Check sheet for the drawn part. Datum: minimum x, y, z corner. Units: mm. A direction names the side the tool comes from. Round coordinates to 2 decimals unless told otherwise and drop trailing zeros. Write each loop counter-clockwise with the first axis right and the second up, starting at its lowest first coordinate (ties: lowest second). Pieces come first, ordered by that corner, then holes. Notation, with made-up numbers: (23.25, -7) - (41.25, -7) arc R11 ccw to (41.25, 7) - close; hole circle Ø1 at (71.5, 29). An arc over 180 degrees is marked (long way). Answer as a JSON object with one key per item and string values. Group by question number.
1) Set-up check for the marked faces 1, 2 and 3: record each of +Z, -Z, +X, -X, +Y, -Y from which the full face is reachable in a straight line by a thin tool's end or side.
2) Section check C-C (x = 66). Enter the section's corners in (y, z), then the cut area to 3 significant figures.
3) Thickness scan on line 1 (Y direction, x = 42, z = 3.75); line 2 (X direction, y = 7.1, z = 63); line 3 (Y direction, x = 66, z = 5). Record the ranges inside material, lowest first.
4) Section check D-D (y = 71). Enter the section's corners in (x, z).
5) Go/stop test with flat-tipped pins: pin 1 Ø3 at (y, z) = (14, 43) entering from -X; pin 2 Ø4 at (x, y) = (20.5, 42.5) entering from +Z; pin 3 Ø16 at (x, z) = (16, 23.5) entering from -Y; pin 4 Ø6.5 at (x, z) = (5, 103) entering from +Y. Record where each tip stops, or that it passes through.
6) Section check B-B (z = 23). Enter the section's corners in (x, y), then the cut area to 3 significant figures.
7) Section check A-A (y = 14). Enter the section's corners in (x, z).
8) Mould release check, pull along Z, two halves, no side actions. Record for the marked faces 4, 5, 6 and 7: +Z half, -Z half, draft (parallel to the pull), parting line (faces both ways), or undercut.
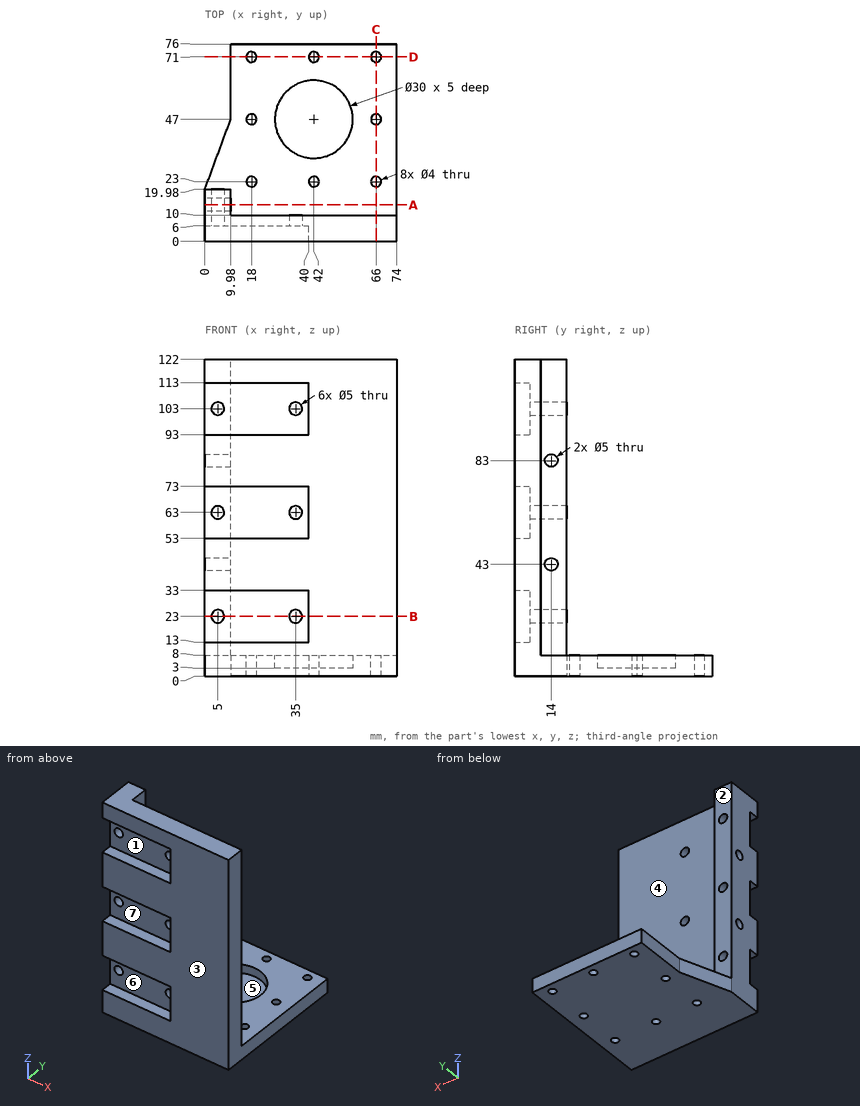
Returned:
{
 "1": {"face 1": "-X, -Y", "face 2": "+Z, +X, -X, +Y", "face 3": "+Z, -Z, +X, -X, -Y"},
 "2": {"outline": "(0, 0) - (21, 0) - (21, 8) - (10, 8) - (10, 122) - (0, 122) - close; (25, 0) - (45, 0) - (45, 8) - (25, 8) - close; (49, 0) - (69, 0) - (69, 8) - (49, 8) - close; (73, 0) - (76, 0) - (76, 8) - (73, 8) - close", "area": "1,650 mm2"},
 "3": {"line 1": "0 to 21, 25 to 32, 62 to 69, 73 to 76", "line 2": "0 to 2.5, 7.5 to 32.5, 37.5 to 74", "line 3": "0 to 21, 25 to 45, 49 to 69, 73 to 76"},
 "4": {"outline": "(9.98, 0) - (16, 0) - (16, 8) - (9.98, 8) - close; (20, 0) - (40, 0) - (40, 8) - (20, 8) - close; (44, 0) - (64, 0) - (64, 8) - (44, 8) - close; (68, 0) - (74, 0) - (74, 8) - (68, 8) - close"},
 "5": {"pin 1": "through", "pin 2": "z = 8", "pin 3": "y = 6", "pin 4": "y = 19.98"},
 "6": {"outline": "(0, 6) - (2.5, 6) - (2.5, 19.98) - (0, 19.98) - close; (7.5, 6) - (32.5, 6) - (32.5, 10) - (9.98, 10) - (9.98, 19.98) - (7.5, 19.98) - close; (37.5, 6) - (40, 6) - (40, 0) - (74, 0) - (74, 10) - (37.5, 10) - close", "area": "510 mm2"},
 "7": {"outline": "(0, 0) - (74, 0) - (74, 8) - (9.98, 8) - (9.98, 40.5) - (0, 40.5) - close; (0, 45.5) - (9.98, 45.5) - (9.98, 80.5) - (0, 80.5) - close; (0, 85.5) - (9.98, 85.5) - (9.98, 122) - (0, 122) - close; hole circle Ø5 at (5, 23); hole circle Ø5 at (5, 63); hole circle Ø5 at (5, 103)"},
 "8": {"face 4": "draft", "face 5": "+Z half", "face 6": "undercut", "face 7": "undercut"}
}
